Verification items for the finished model (mm, model axes). A direction names the side the tool comes from. Coordinates: 2 decimals unless noted, no trailing zeros. Loops run counter-clockwise (first coordinate to the right, second up) from the corner with the lowest first, then second, coordinate; pieces in that order, holes last. Notation, with made-up numbers: M -30,82.25 L -11,82.25 A21 ccw -11,87.25 Z; hole C 68,-16 d10. An arc over 180 degrees is marked long. Write item = value, one per line. Start each with the question number.
```python
from build123d import *

# Parameters (mm, degrees)
SKIZZE1_R                            = 6
AUFSATZ_LINEAR_AUSTRAGEN1_DEPTH      = 3.25
SCHNITT_LINEAR_AUSTRAGEN1_DEPTH      = 10.086390923
VERRUNDUNG2_R                        = 0.3
KREISMUSTER1_START                   = -3.25
KREISMUSTER1_DEPTH                   = 6.5
SCHNITT_LINEAR_AUSTRAGEN2_DEPTH      = 10.068181427
SCHNITT_LINEAR_AUSTRAGEN2_DEPTH_BACK = 10.068181427


# Read off the part's stored shape, not the designer's step: Kreismuster1
with BuildPart() as part:
    # Skizze1 → Aufsatz-Linear austragen1 (new, symmetric)
    with BuildSketch(Plane.XY):
        with Locations(Location((0, 0, 0), (0, 0, 180))):
            Circle(SKIZZE1_R)
    extrude(amount=AUFSATZ_LINEAR_AUSTRAGEN1_DEPTH, both=True)

    # Skizze2 → Schnitt-Linear austragen1 (cut, symmetric)
    with BuildSketch(Plane.XY):
        with BuildLine():
            Line((0.95, 5.75), (0.95, 6))
            Line((0.95, 6), (-0.95, 6))
            Line((-0.95, 6), (-0.95, 5.75))
            ThreePointArc((-0.95, 5.75), (0, 4.8), (0.95, 5.75))
        make_face()
    extrude(amount=SCHNITT_LINEAR_AUSTRAGEN1_DEPTH, both=True, mode=Mode.SUBTRACT)

    # Verrundung2
    verrundung2_edges = [part.edges().sort_by_distance(p)[0] for p in [
        (0.95, 5.924314306, 0),
        (-0.95, 5.924314306, 0),
    ]]
    fillet(verrundung2_edges, radius=VERRUNDUNG2_R)

    # Kreismuster1 outline → Kreismuster1 (cut)
    with BuildSketch(Plane.XY.offset(KREISMUSTER1_START)):
        with BuildLine():
            ThreePointArc((1.301196241, 5.857208238), (1.4202728, 5.709694635), (1.427132072, 5.520241632))
            ThreePointArc((1.427132072, 5.520241632), (1.945632522, 4.388033855), (3.139589709, 4.741874783))
            ThreePointArc((3.139589709, 4.741874783), (3.337990982, 4.875510752), (3.571043132, 4.821581789))
            ThreePointArc((3.571043132, 4.821581789), (2.49054405, 5.458680274), (1.301196241, 5.857208238))
        make_face()
        with BuildLine():
            ThreePointArc((-1.301196241, 5.857208238), (-2.440419859, 5.481272746), (-3.482083764, 4.886214553))
            ThreePointArc((-3.482083764, 4.886214553), (-3.292782023, 4.875999815), (-3.147401255, 4.754328445))
            ThreePointArc((-3.147401255, 4.754328445), (-1.952335887, 4.385018197), (-1.427132072, 5.520241632))
            ThreePointArc((-1.427132072, 5.520241632), (-1.4202728, 5.709694635), (-1.301196241, 5.857208238))
        make_face()
        with BuildLine():
            ThreePointArc((-3.482083764, 4.886214553), (-4.421893009, 4.055473119), (-5.168444311, 3.047488049))
            ThreePointArc((-5.168444311, 3.047488049), (-4.991353857, 3.115152376), (-4.809053712, 3.063131734))
            ThreePointArc((-4.809053712, 3.063131734), (-3.572034677, 3.206383521), (-3.539604337, 4.451247144))
            ThreePointArc((-3.539604337, 4.451247144), (-3.60539033, 4.681233753), (-3.482083764, 4.886214553))
        make_face()
        with BuildLine():
            ThreePointArc((-5.168444311, 3.047488049), (-5.689109795, 1.906313128), (-5.961133882, 0.681823175))
            ThreePointArc((-5.961133882, 0.681823175), (-5.826875264, 0.815666791), (-5.639177093, 0.842291719))
            ThreePointArc((-5.639177093, 0.842291719), (-4.567369724, 1.476299708), (-5.044074785, 2.626729824))
            ThreePointArc((-5.044074785, 2.626729824), (-5.197717262, 2.810075472), (-5.168444311, 3.047488049))
        make_face()
        with BuildLine():
            ThreePointArc((-5.961133882, 0.681823175), (-5.972627813, -0.572465721), (-5.72308925, -1.801735119))
            ThreePointArc((-5.72308925, -1.801735119), (-5.654877001, -1.624854993), (-5.494235524, -1.524188187))
            ThreePointArc((-5.494235524, -1.524188187), (-4.772965052, -0.509049737), (-5.676378878, 0.348027053))
            ThreePointArc((-5.676378878, 0.348027053), (-5.891311659, 0.453029612), (-5.961133882, 0.681823175))
        make_face()
        with BuildLine():
            ThreePointArc((-5.72308925, -1.801735119), (-5.223424224, -2.952260046), (-4.495470494, -3.973757043))
            ThreePointArc((-4.495470494, -3.973757043), (-4.505099133, -3.784424586), (-4.39929072, -3.627122108))
            ThreePointArc((-4.39929072, -3.627122108), (-4.153271361, -2.406379857), (-5.327185496, -1.990852756))
            ThreePointArc((-5.327185496, -1.990852756), (-5.566244749, -1.982349183), (-5.72308925, -1.801735119))
        make_face()
        with BuildLine():
            ThreePointArc((-4.495470494, -3.973757043), (-3.571043132, -4.821581789), (-2.490544049, -5.458680274))
            ThreePointArc((-2.490544049, -5.458680274), (-2.576348697, -5.289632788), (-2.543668584, -5.102893665))
            ThreePointArc((-2.543668584, -5.102893665), (-2.815439322, -3.887625039), (-4.056873345, -3.985496038))
            ThreePointArc((-4.056873345, -3.985496038), (-4.278723555, -4.074961795), (-4.495470494, -3.973757043))
        make_face()
        with BuildLine():
            ThreePointArc((-2.490544049, -5.458680274), (-1.301196241, -5.857208238), (-0.054979913, -5.999748095))
            ThreePointArc((-0.054979913, -5.999748095), (-0.202124166, -5.880215427), (-0.248223041, -5.69632855))
            ThreePointArc((-0.248223041, -5.69632855), (-0.990792245, -4.696664534), (-2.085090937, -5.291010847))
            ThreePointArc((-2.085090937, -5.291010847), (-2.251372186, -5.462976493), (-2.490544049, -5.458680274))
        make_face()
        with BuildLine():
            ThreePointArc((-0.054979913, -5.999748095), (1.193639301, -5.880070171), (2.39009075, -5.503404965))
            ThreePointArc((2.39009075, -5.503404965), (2.20704947, -5.454055398), (2.090142521, -5.304816478))
            ThreePointArc((2.090142521, -5.304816478), (1.005171811, -4.693608063), (0.247222636, -5.681661814))
            ThreePointArc((0.247222636, -5.681661814), (0.165261886, -5.906392926), (-0.054979913, -5.999748095))
        make_face()
        with BuildLine():
            ThreePointArc((2.39009075, -5.503404965), (3.482083764, -4.886214553), (4.421893009, -4.055473119))
            ThreePointArc((4.421893009, -4.055473119), (4.234604202, -4.084839642), (4.067103452, -3.996053445))
            ThreePointArc((4.067103452, -3.996053445), (2.82733253, -3.878984118), (2.53678917, -5.089901837))
            ThreePointArc((2.53678917, -5.089901837), (2.553320677, -5.328540364), (2.39009075, -5.503404965))
        make_face()
        with BuildLine():
            ThreePointArc((4.421893009, -4.055473119), (5.168444311, -3.047488049), (5.689109795, -1.906313128))
            ThreePointArc((5.689109795, -1.906313128), (5.529957397, -2.009318003), (5.340825248, -1.996336468))
            ThreePointArc((5.340825248, -1.996336468), (4.160621768, -2.393648579), (4.38772181, -3.618051592))
            ThreePointArc((4.38772181, -3.618051592), (4.499887126, -3.829334765), (4.421893009, -4.055473119))
        make_face()
        with BuildLine():
            ThreePointArc((5.689109795, -1.906313128), (5.961133882, -0.681823176), (5.972627814, 0.572465721))
            ThreePointArc((5.972627814, 0.572465721), (5.86913072, 0.413632974), (5.691069839, 0.34856522))
            ThreePointArc((5.691069839, 0.34856522), (4.774501705, -0.494429456), (5.479977488, -1.520607358))
            ThreePointArc((5.479977488, -1.520607358), (5.668382211, -1.668002397), (5.689109795, -1.906313128))
        make_face()
        with BuildLine():
            ThreePointArc((5.972627814, 0.572465721), (5.72308925, 1.801735119), (5.223424223, 2.952260047))
            ThreePointArc((5.223424223, 2.952260047), (5.193478023, 2.765063051), (5.057276753, 2.633196816))
            ThreePointArc((5.057276753, 2.633196816), (4.562826922, 1.490281013), (5.624695274, 0.839763703))
            ThreePointArc((5.624695274, 0.839763703), (5.856762517, 0.78174274), (5.972627814, 0.572465721))
        make_face()
        with BuildLine():
            ThreePointArc((5.223424223, 2.952260047), (4.495470494, 3.973757044), (3.571043132, 4.821581789))
            ThreePointArc((3.571043132, 4.821581789), (3.619825794, 4.638388607), (3.549034572, 4.462524759))
            ThreePointArc((3.549034572, 4.462524759), (3.562197912, 3.217308355), (4.796852148, 3.05493199))
            ThreePointArc((4.796852148, 3.05493199), (5.032455375, 3.096317454), (5.223424223, 2.952260047))
        make_face()
    extrude(amount=KREISMUSTER1_DEPTH, mode=Mode.SUBTRACT)

    # Skizze3 → Schnitt-Linear austragen2 (cut, two sides: drawn at the far end of the back side and taken through both)
    with BuildSketch(Plane.XY.offset(-SCHNITT_LINEAR_AUSTRAGEN2_DEPTH_BACK)):
        with BuildLine():
            Line((1.549193338, 2.15), (-1.549193338, 2.15))
            ThreePointArc((-1.549193338, 2.15), (0, -2.65), (1.549193338, 2.15))
        make_face()
    extrude(amount=SCHNITT_LINEAR_AUSTRAGEN2_DEPTH + SCHNITT_LINEAR_AUSTRAGEN2_DEPTH_BACK, mode=Mode.SUBTRACT)


solid = part.part
```
Q1. Scan lines: L1, parallel to Y at x = 5, z = -0.5; L2, parallel to Y at x = 0, z = 0.5; L3, parallel to Y at x = -0.75, z = -0.5. Record each from-to range of solid material in increasing order. Write a range as [from, to].
Q2. Set-up check for faces 1 (the face through (1.928, 4.396, -0.046)), 2 (the face through (-4.77, -0.53, -0.05)): record each of +Z, -Z, +X, -X, +Y, -Y from which the full face is reachable in a straight line by a thin tool's end or side.
Q3. Gauge pin test, flat ends, axial feed: pin 1 (6 mm diameter, centred on x = 0, y = 0, fed in from -Z); pin 2 (1 mm diameter, centred on x = -4.5, z = 1, fed in from -Y); pin 3 (1.5 mm diameter, centred on y = 2, z = 1.5, fed in from +X). Record the tip position at first contact, or that the pin passes through.
Q4. Sectioned sample at B-B on x = -0.75. Record the cut outline in (y, z), plus the area to 3 significant figures.
Q5. Sectioned sample at A-A on y = 1. Record the cut outline in (x, z).
Q6. Mould release check, pull along Y, two halves, no side actions. Record for faces 3 (the face through (0.1, 2.5, 3.25)), 4 (the face through (4.777, -0.476, -0.046)), 5 (the face through (0, 4.8, 0)): +Y half, -Y half, draft (parallel to the pull), parting line (faces both ways), or undercut.
Solutions:
q1.L1 = [-1.93, -1.22], [0.02, 0.95], [2.6, 3.1]
q1.L2 = [-6, -2.65], [2.15, 4.8]
q1.L3 = [-4.79, -2.54], [2.15, 5.17]
q2.face_1 = +Z, -Z
q2.face_2 = +Z, -Z, -X
q3.pin_1 = -3.25
q3.pin_2 = -4.08
q3.pin_3 = 5.19
q4.outline = M -4.79,-3.25 L -2.54,-3.25 L -2.54,3.25 L -4.79,3.25 Z; M 2.15,-3.25 L 5.17,-3.25 L 5.17,3.25 L 2.15,3.25 Z
q4.area = 34.2 mm²
q5.outline = M -4.92,-3.25 L -2.45,-3.25 L -2.45,3.25 L -4.92,3.25 Z; M 2.45,-3.25 L 4.92,-3.25 L 4.92,3.25 L 2.45,3.25 Z
q6.face_3 = draft
q6.face_4 = undercut
q6.face_5 = +Y half
